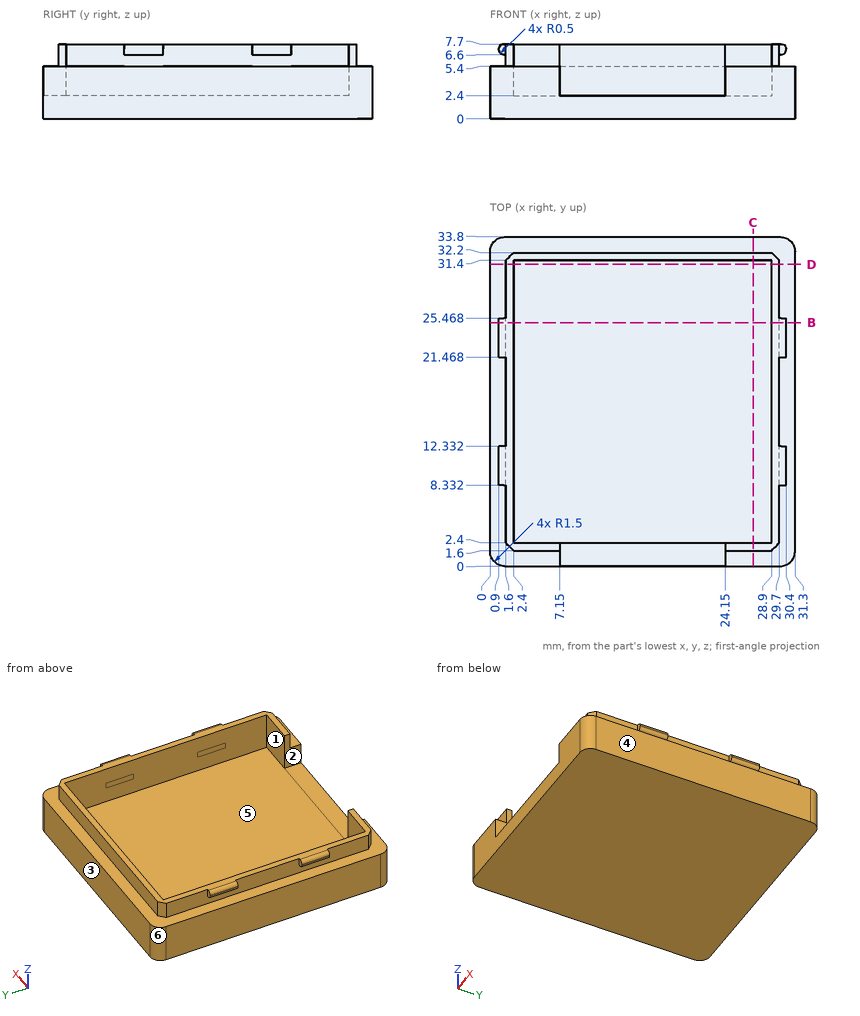
Study the drawing (mm; zero at the part's minimum x, y, z) and answer. A direction names the side the tool comes from. Give positions to 0.01 mm unless a question says otherwise; leave off trailing zeros. Write each loop counter-clockwise with the first axis right and the second up, starting at its lowest first coordinate (ties: lowest second). Pieces come first, ordered by that corner, then holes. Notation, with made-up numbers: (-37, -12) - (-14, -12) arc R17 cw to (-14, 16) - close; hole circle Ø4 at (-38, 14.25). An arc over 180 degrees is marked (long way). Use CSV: the item, a comma, the result in double quotes. Start each with the question number.
(1) Find section D-D (y = 31). Give the vertices of the cut face in (x, z), plus the area to 3 significant figures.
(2) Given P1, Ø0.7, axis at x = 6, z = 6, coming from the -Y side; P2, Ø1.8, axis at y = 14, z = 6, coming from the +X side; P3, Ø0.8, axis at x = 1.5, z = 7, coming from the -Y side, each flat-ended and moving along its own axis, determine where each tip first touches the part or whether it passes through.
(3) For the marked faces 1, 2 and 3, determine the directions among +Z, -Z, +X, -X, +Y, -Y from which every point of the face is accessible in a straight line to the end or side of a thin tool.
(4) Find section B-B (y = 25). Give the vertices of the cut face in (x, z).
(5) Determine the mould class of the marked faces 4, 5 and 6 for opening direction Y: +Y half, -Y half, draft (parallel to the pull), parting line (faces both ways), or undercut.
(6) Consider line 1 along X through (y, z) = (7, 3.5); line 2 along Y through (x, z) = (4, 3.25); line 3 along X through (y, z) = (26, 6.25). Determine where each line is inside the solid, lowest interval first.
(7) Find section C-C (x = 27). Give the vertices of the cut face in (y, z), plus the area to 3 significant figures.
Findings below:
1,outline,"(0, 0) - (31.3, 0) - (31.3, 5.4) - (29.7, 5.4) - (29.7, 7.7) - (28.9, 7.7) - (28.9, 2.4) - (2.4, 2.4) - (2.4, 7.7) - (1.6, 7.7) - (1.6, 5.4) - (0, 5.4) - close"
1,area,"93.2 mm2"
2,P1,"y = 1.6"
2,P2,"x = 31.3"
2,P3,"y = 2.1"
3,face 1,"+Z"
3,face 2,"+Z, -Y"
3,face 3,"+Z, -Z, +X, -X, +Y"
4,outline,"(0, 0) - (31.3, 0) - (31.3, 5.4) - (29.7, 5.4) - (29.7, 6.6) - (29.9, 6.6) arc R0.5 ccw to (30.4, 7.1) - (30.4, 7.2) arc R0.5 ccw to (29.9, 7.7) - (28.9, 7.7) - (28.9, 5.4) - (28.9, 2.4) - (2.4, 2.4) - (2.4, 7.7) - (1.4, 7.7) arc R0.5 ccw to (0.9, 7.2) - (0.9, 7.1) arc R0.5 ccw to (1.4, 6.6) - (1.6, 6.6) - (1.6, 5.4) - (0, 5.4) - close"
5,face 4,"draft"
5,face 5,"undercut"
5,face 6,"+Y half"
6,line 1,"0 to 2.4, 28.9 to 31.3"
6,line 2,"0 to 2.4, 31.4 to 33.8"
6,line 3,"1.6 to 2.4, 28.9 to 29.7"
7,outline,"(0, 0) - (33.8, 0) - (33.8, 5.4) - (32.2, 5.4) - (32.2, 7.7) - (31.4, 7.7) - (31.4, 2.4) - (2.4, 2.4) - (2.4, 7.7) - (1.6, 7.7) - (1.6, 5.4) - (0, 5.4) - close"
7,area,"99.2 mm2"
